```python
from build123d import *

# Parameters (mm, degrees)
SKETCH1_W                  = 25.4
SKETCH1_H                  = 1498.6
BOSS_EXTRUDE1_DEPTH        = 25.4
SKETCH2_W                  = 23.114
SKETCH2_H                  = 23.114
CUT_EXTRUDE1_DEPTH         = 1499.6
M3_5_CLEARANCE_HOLE1_D     = 4.1402
M3_5_CLEARANCE_HOLE1_DEPTH = 25.4
M3_5_CLEARANCE_HOLE2_D     = 4.1402
M3_5_CLEARANCE_HOLE2_DEPTH = 25.4
CHAMFER1_SIZE              = 2.159
FILLET1_R                  = 0.8128
FILLET2_R                  = 3.0988
SKETCH8_W                  = 95.882963774
SKETCH8_H                  = 79.338329604
CUT_EXTRUDE3_DEPTH         = 1371.6


with BuildPart() as part:
    # Sketch1 → Boss-Extrude1 (new body)
    with BuildSketch(Plane(origin=(0, 0, 0), x_dir=(0, -1, 0), z_dir=(-1, 0, 0))):
        with Locations((-12.7, 0)):
            Rectangle(SKETCH1_W, SKETCH1_H)
    extrude(amount=-BOSS_EXTRUDE1_DEPTH)

    # Sketch2 → Cut-Extrude1 (cut, through all)
    with BuildSketch(Plane(origin=(0, 0, -749.3), x_dir=(-1, 0, 0), z_dir=(0, 0, -1))):
        with Locations((-13.843, 13.843)):
            Rectangle(SKETCH2_W, SKETCH2_H)
    extrude(amount=-CUT_EXTRUDE1_DEPTH, mode=Mode.SUBTRACT)

    # M3.5 Clearance Hole1
    with Locations(Plane(origin=(0, 0, 0), x_dir=(-1, 0, 0), z_dir=(0, -1, 0))):
        with Locations((-12.7, 736.6), (-12.7, 711.2), (-12.7, 685.8), (-12.7, 660.4), (-12.7, 635), (-12.7, 609.6), (-12.7, 584.2), (-12.7, 558.8), (-12.7, 533.4), (-12.7, 508), (-12.7, 482.6), (-12.7, 457.2), (-12.7, 431.8), (-12.7, 406.4), (-12.7, 381), (-12.7, 355.6), (-12.7, 330.2), (-12.7, 304.8), (-12.7, 279.4), (-12.7, 254), (-12.7, 228.6), (-12.7, 203.2), (-12.7, 177.8), (-12.7, 152.4), (-12.7, 127), (-12.7, 101.6), (-12.7, 76.2), (-12.7, 50.8), (-12.7, 25.4), (-12.7, 0), (-12.7, -25.4), (-12.7, -50.8), (-12.7, -76.2), (-12.7, -101.6), (-12.7, -127), (-12.7, -152.4), (-12.7, -177.8), (-12.7, -203.2), (-12.7, -228.6), (-12.7, -254), (-12.7, -279.4), (-12.7, -304.8), (-12.7, -330.2), (-12.7, -355.6), (-12.7, -381), (-12.7, -406.4), (-12.7, -431.8), (-12.7, -457.2), (-12.7, -482.6), (-12.7, -508), (-12.7, -533.4), (-12.7, -558.8), (-12.7, -584.2), (-12.7, -609.6), (-12.7, -635), (-12.7, -660.4), (-12.7, -685.8), (-12.7, -711.2), (-12.7, -736.6)):
            Hole(M3_5_CLEARANCE_HOLE1_D / 2, depth=M3_5_CLEARANCE_HOLE1_DEPTH)

    # M3.5 Clearance Hole2
    with Locations(Plane.ZY):
        with Locations((711.2, 12.7), (736.6, 12.7), (685.8, 12.7), (660.4, 12.7), (635, 12.7), (609.6, 12.7), (584.2, 12.7), (558.8, 12.7), (533.4, 12.7), (508, 12.7), (482.6, 12.7), (457.2, 12.7), (431.8, 12.7), (406.4, 12.7), (381, 12.7), (355.6, 12.7), (330.2, 12.7), (304.8, 12.7), (279.4, 12.7), (254, 12.7), (228.6, 12.7), (203.2, 12.7), (177.8, 12.7), (152.4, 12.7), (127, 12.7), (101.6, 12.7), (76.2, 12.7), (50.8, 12.7), (25.4, 12.7), (0, 12.7), (-25.4, 12.7), (-50.8, 12.7), (-76.2, 12.7), (-101.6, 12.7), (-127, 12.7), (-152.4, 12.7), (-177.8, 12.7), (-203.2, 12.7), (-228.6, 12.7), (-254, 12.7), (-279.4, 12.7), (-304.8, 12.7), (-330.2, 12.7), (-355.6, 12.7), (-381, 12.7), (-406.4, 12.7), (-431.8, 12.7), (-457.2, 12.7), (-482.6, 12.7), (-508, 12.7), (-533.4, 12.7), (-558.8, 12.7), (-584.2, 12.7), (-609.6, 12.7), (-635, 12.7), (-660.4, 12.7), (-685.8, 12.7), (-711.2, 12.7), (-736.6, 12.7)):
            Hole(M3_5_CLEARANCE_HOLE2_D / 2, depth=M3_5_CLEARANCE_HOLE2_DEPTH)

    # Chamfer1
    chamfer1_edges = [part.edges().sort_by_distance(p)[0] for p in [
        (25.4, 1.143, -749.3),
        (1.143, 25.4, 749.3),
        (1.143, 25.4, -749.3),
        (25.4, 1.143, 749.3),
    ]]
    chamfer(chamfer1_edges, length=CHAMFER1_SIZE)

    # Fillet1
    fillet1_edges = [part.edges().sort_by_distance(p)[0] for p in [
        (2.286, 2.286, 0),
    ]]
    fillet(fillet1_edges, radius=FILLET1_R)

    # Fillet2
    fillet2_edges = [part.edges().sort_by_distance(p)[0] for p in [
        (0, 0, 0),
    ]]
    fillet(fillet2_edges, radius=FILLET2_R)

    # Sketch8 → Cut-Extrude3 (cut)
    with BuildSketch(Plane.XY.offset(749.3)):
        with Locations((2.286, 3.0988)):
            Rectangle(SKETCH8_W, SKETCH8_H)
    extrude(amount=-CUT_EXTRUDE3_DEPTH, mode=Mode.SUBTRACT)


solid = part.part
```
Model file for the job. Use its own axes, mm. A direction names the side the tool comes from. Coordinates: 2 decimals unless noted, no trailing zeros. Loops run counter-clockwise (first coordinate to the right, second up) from the corner with the lowest first, then second, coordinate; pieces in that order, holes last. Notation, with made-up numbers: M 47.5,23.25 L 96.5,23.25 A17 cw 96.5,46.25 Z; hole C -9.75,-20.5 d2. An arc over 180 degrees is marked long. Use CSV: the item, a comma, the result in double quotes. Start each with the question number.
1. Two-plate mould, pull along Z, no slides. Class faces 3 (the cylindrical face through (1.159, 13.322, -662.375)), 4 (the flat face through (17, 0, -687)), 5 (the flat face through (2, 8, -749.3)): pulls with the +Z half, pulls with the -Z half, needs draft (parallel to the pull), parting line crosses it, or undercut.
2. Band-saw the part on B-B, the plane z = -685.8. List the corners of the cut face in (x, y).
3. Probe probe 1 along Z at (x, y) = (12.7, 0.55); probe 2 along X at (y, z) = (18.25, -733.5). List the from-to ranges inside material, lowest first. Write a range as [from, to].
4. Band-saw the part on D-D, the plane z = -656. List the corners of the cut face in (x, y), then the cut area to 3 significant figures.
5. Band-saw the part on A-A, the plane y = 12.7. List the corners of the cut face in (x, z), then the cut area to 3 significant figures.
6. Tool access for faces 1 (the flat face through (2.286, 17, -687)), 2 (the cylindrical face through (12.25, 1.16, -734.58)): list every direction of +Z, -Z, +X, -X, +Y, -Y with a clear straight run to the whole face (end or side of a thin tool).
7. Flat gauge pins, fed straight in: pin 1 (6.5 mm diameter, centred on x = 12.7, z = -711.2, fed in from +Y); pin 2 (5 mm diameter, centred on y = 12.7, z = -711.2, fed in from -X); pin 3 (12 mm diameter, centred on y = 10.5, z = -716.5, fed in from +X). Where does each tip first touch, or does it go through?
Entries:
1,face 3,"undercut"
1,face 4,"needs draft"
1,face 5,"pulls with the -Z half"
2,outline,"M 0,3.1 A3.1 ccw 3.1,0 L 10.63,0 L 10.63,2.29 L 3.1,2.29 A0.81 cw 2.29,3.1 L 2.29,10.63 L 0,10.63 Z; M 0,14.77 L 2.29,14.77 L 2.29,25.4 L 0,25.4 Z; M 14.77,0 L 25.4,0 L 25.4,2.29 L 14.77,2.29 Z"
3,probe 1,"z = [-749.3, -738.67], [-734.53, -713.27], [-709.13, -687.87], [-683.73, -662.47], [-658.33, -637.07], [-632.93, -622.3]"
3,probe 2,"x = [0, 2.29]"
4,outline,"M 0,3.1 A3.1 ccw 3.1,0 L 25.4,0 L 25.4,2.29 L 3.1,2.29 A0.81 cw 2.29,3.1 L 2.29,25.4 L 0,25.4 Z"
4,area,"109 mm2"
5,outline,"M 0,-749.3 L 2.29,-749.3 L 2.29,-738.67 L 0,-738.67 Z; M 0,-734.53 L 2.29,-734.53 L 2.29,-713.27 L 0,-713.27 Z; M 0,-709.13 L 2.29,-709.13 L 2.29,-687.87 L 0,-687.87 Z; M 0,-683.73 L 2.29,-683.73 L 2.29,-662.47 L 0,-662.47 Z; M 0,-658.33 L 2.29,-658.33 L 2.29,-637.07 L 0,-637.07 Z; M 0,-632.93 L 2.29,-632.93 L 2.29,-622.3 L 0,-622.3 Z"
5,area,"243 mm2"
6,face 1,"+Z, -Z, +X, +Y"
6,face 2,"+Y, -Y"
7,pin 1,"stops at y = 2.29"
7,pin 2,"stops at x = 0"
7,pin 3,"stops at x = 2.29"
